```python
from build123d import *

# Parameters (mm, degrees)
BOSS_EXTRUDE3_DEPTH      = 1
BOSS_EXTRUDE3_DEPTH_BACK = 1.791091685
CUT_EXTRUDE4_DEPTH       = 134.344317451
CUT_EXTRUDE7_DEPTH       = 134.344317451


with BuildPart() as part:
    # Sketch2 → Boss-Extrude3 (new, two sides: drawn at the far end of the back side and taken through both)
    with BuildSketch(Plane(origin=(0, 39.78932127, 0), x_dir=(1, 0, 0), z_dir=(0, 1, 0)).offset(-BOSS_EXTRUDE3_DEPTH_BACK)):
        with BuildLine():
            Line((-62.934827524, 31.1490062), (-36.827019598, 82.334560695))
            Line((-36.827019598, 82.334560695), (-58.206533771, 93.239439133))
            Line((-58.206533771, 93.239439133), (-95.285485747, 14.655800367))
            ThreePointArc((-95.285485747, 14.655800367), (-81.079538231, 26.765253936), (-62.934827524, 31.1490062))
        make_face()
    extrude(amount=BOSS_EXTRUDE3_DEPTH + BOSS_EXTRUDE3_DEPTH_BACK)

    # Sketch14 → Cut-Extrude4 (cut, through all)
    with BuildSketch(Plane(origin=(0, 40.78932127, 0), x_dir=(1, 0, 0), z_dir=(0, 1, 0))):
        Polygon((-60.497453494, 77.385579161), (-49.198590392, 71.186677889), (-43.491580172, 81.777523219), (-54.878158967, 87.916549938), align=None)
    extrude(amount=-CUT_EXTRUDE4_DEPTH, mode=Mode.SUBTRACT)

    # Sketch15 → Cut-Extrude7 (cut, through all)
    with BuildSketch(Plane(origin=(0, 40.78932127, 0), x_dir=(1, 0, 0), z_dir=(0, 1, 0))):
        with BuildLine():
            Line((-69.15808426, 59.503123178), (-57.079111782, 54.0598094))
            Line((-57.079111782, 54.0598094), (-62.805804845, 42.724997947))
            Line((-62.805804845, 42.724997947), (-74.883268234, 48.631494641))
            ThreePointArc((-74.883268234, 48.631494641), (-71.899649138, 54.003573981), (-69.15808426, 59.503123178))
        make_face()
    extrude(amount=-CUT_EXTRUDE7_DEPTH, mode=Mode.SUBTRACT)


solid = part.part
```
Geometry: final body of the model. Coordinates: model frame, mm. A direction names the side the tool comes from. Coordinates: 2 decimals unless noted, no trailing zeros. Order: outer loops, then holes, each group sorted by start corner. A loop starts at its lowest first (then second) coordinate and runs counter-clockwise, first axis right, second up. Notation, with made-up numbers: (20.25, 3) - (29.25, 3) arc R23 cw to (29.25, 21) - close; hole circle Ø9 at (-2.5, 18). An arc over 180 degrees is marked (long way). Return JSON: item names as keys, results as strings. Group by question number.
1. Cut plane B-B (x = -65). Output: boundary loops of the cut face in (y, z), plus the area to 3 significant figures.
2. Cut plane C-C (z = -86). Output: boundary loops of the cut face in (x, y).
3. Set-up query: faces 5 (the face through (-54.93, 39.41, -74.33)), 6 (the face through (-62, 37.998, -57)). Return all of +Z, -Z, +X, -X, +Y, -Y with unobstructed straight access to the full face (end or side cutting, diameter ignored); none if empty.
4. Material intervals for line 1 along X through (y, z) = (40.2, -57); line 2 along Z through (x, y) = (-64.5, 39.95); line 3 along Z through (x, y) = (-57.5, 38.2), sorted ascending. Write a range as [from, to].
5. Cut plane D-D (z = -19.5). Output: boundary loops of the cut face in (x, y).
6. Pull-direction query (Z, two-part tool) for faces 1 (the face through (-49.1, 39.4, -84.8)), 2 (the face through (-47.37, 39.37, -87.71)), 3 (the face through (-46.385, 39.413, -76.408)), 4 (the face through (-62, 40.789, -57)); classes: pulls with the +Z half, pulls with the -Z half, needs draft (parallel to the pull), parting line crosses it, or undercut.
7. Cut plane A-A (y = 38.8). Output: boundary loops of the cut face in (x, z) (1 decimal), plus the area to 3 significant figures.
Resolved:
{
 "1": {"outline": "(38, -78.84) - (40.79, -78.84) - (40.79, -57.63) - (38, -57.63) - close; (38, -43.8) - (40.79, -43.8) - (40.79, -31.09) - (38, -31.09) - close", "area": "94.7 mm²"},
 "2": {"outline": "(-61.62, 38) - (-55.9, 38) - (-55.9, 40.79) - (-61.62, 40.79) - close; (-51.32, 38) - (-44.01, 38) - (-44.01, 40.79) - (-51.32, 40.79) - close"},
 "3": {"face 5": "+Y, -Y", "face 6": "+Z, -Z, +X, -X, -Y"},
 "4": {"line 1": "x = [-75.31, -70.37], [-63.6, -49.75]", "line 2": "z = [-79.9, -57.4], [-43.55, -31.11]", "line 3": "z = [-92.88, -83], [-75.74, -54.25], [-53.23, -41.8]"},
 "5": {"outline": "(-93, 38) - (-91.12, 38) - (-91.12, 40.79) - (-93, 40.79) - close"},
 "6": {"face 1": "undercut", "face 2": "pulls with the -Z half", "face 3": "undercut", "face 4": "needs draft"},
 "7": {"outline": "(-95.3, -14.7) - (-58.2, -93.2) - (-36.8, -82.3) - (-62.9, -31.1) arc R40.2 cw to start; hole (-74.9, -48.6) arc R138 cw to (-69.2, -59.5) - (-57.1, -54.1) - (-62.8, -42.7) - close; hole (-60.5, -77.4) - (-54.9, -87.9) - (-43.5, -81.8) - (-49.2, -71.2) - close", "area": "1,230 mm²"}
}
